Part print with two shaded views. Sizes in mm from the minimum x, y, z corner. Round coordinates to 2 decimals unless told otherwise and drop trailing zeros. Order: outer loops, then holes, each group sorted by start corner. A loop starts at its lowest first (then second) coordinate and runs counter-clockwise, first axis right, second up. Notation, with made-up numbers: (75.25, -1.75) - (86.25, -1.75) arc R25 cw to (86.25, 30.25) - close; hole circle Ø3 at (37, 49). An arc over 180 degrees is marked (long way). Use one line per item in the form item = value.
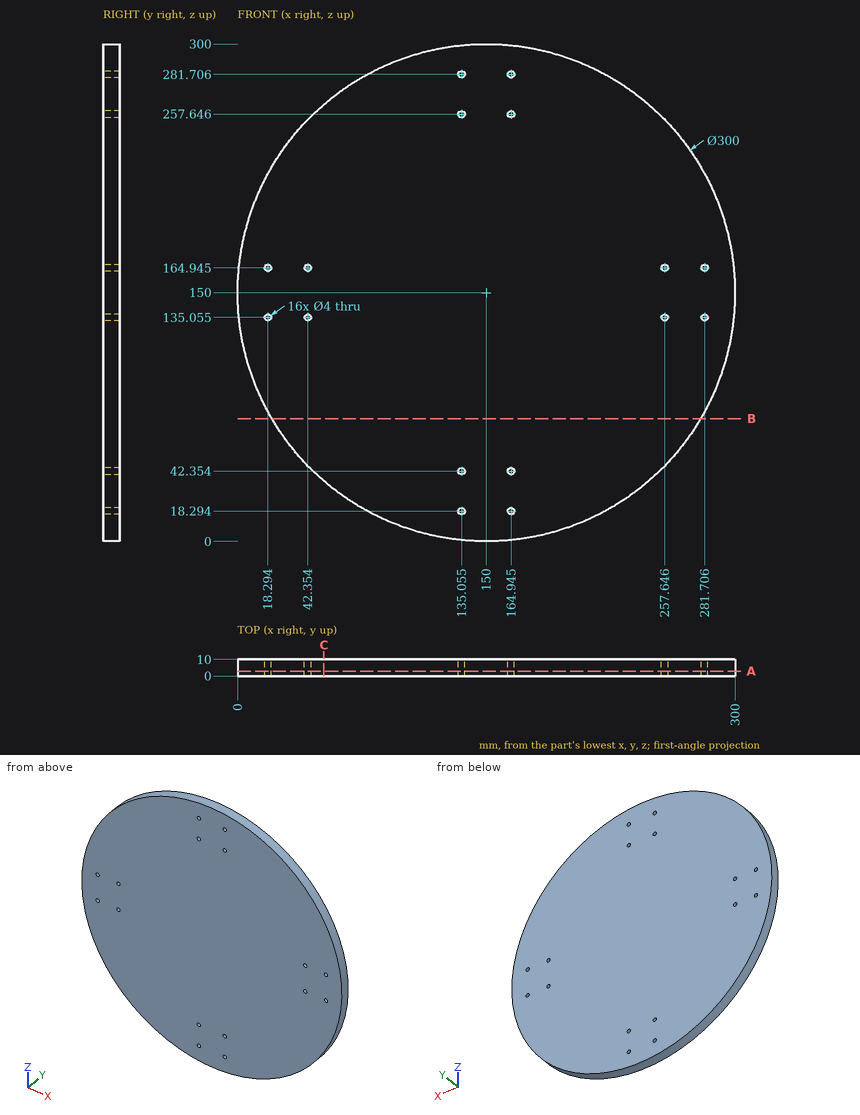
(1) Pin check, flat tips, straight feed: pin 1 (3.5 mm diameter, centred on x = 164.94, z = 281.71, fed in from +Y); pin 2 (6 mm diameter, centred on x = 73, y = 4.5, fed in from +Z) (1 decimal); pin 3 (2 mm diameter, centred on x = 42, y = 2, fed in from -Z) (1 decimal); pin 4 (6 mm diameter, centred on y = 3, z = 115.5, fed in from +X) (1 decimal). Stop position of each tip, or through.
Report:
pin_1 = through
pin_2 = 280.5
pin_3 = 44.9
pin_4 = 296.7
(2) Probe probe 1 along X at (y, z) = (4, 148.5); probe 2 along X at (y, z) = (1.5, 196.5); probe 3 along Z at (x, y) = (181, 8). List the from-to ranges inside material, lowest first. Write a range as [from, to].
Report:
probe_1 = [0.01, 299.99]
probe_2 = [7.39, 292.61]
probe_3 = [3.24, 296.76]
(3) Slice it at C-C on x = 52. Give the cut face in (y, z).
Report:
outline = (0, 36.44) - (10, 36.44) - (10, 263.56) - (0, 263.56) - close
(4) Slice it at B-B on z = 74. Give the cut face in (x, y).
Report:
outline = (20.68, 0) - (279.32, 0) - (279.32, 10) - (20.68, 10) - close
(5) Slice it at A-A on y = 3. Count the separate pieces of the cut face and the enclosed holes in it, then the cut area to 3 significant figures.
Report:
separate_pieces = 1
enclosed_holes = 16
area = 70,500 mm2
